Can you work these out from the model? Positions are in its coordinate system, mm. Give positions to 0.01 mm unless a question says otherwise; leave off trailing zeros. Loops run counter-clockwise (first coordinate to the right, second up) from the corner with the lowest first, then second, coordinate; pieces in that order, holes last. Notation, with made-up numbers: M 53,-29 L 73,-29 A30 cw 73,9 Z; hole C 73,-19 d3. An arc over 180 degrees is marked long. Answer as a JSON object with one key per item and string values.
```python
from build123d import *

# Parameters (mm, degrees)
CUT_EXTRUDE1_DEPTH     = 1.5625
CUT_SWEEP1_PITCH       = 0.8
CUT_SWEEP1_HEIGHT      = 6.05
CUT_SWEEP1_RADIUS      = 2.5
CUT_SWEEP1_START_ANGLE = -90


with BuildPart() as part:
    # Sketch2 → Revolve1 (revolve)
    with BuildSketch(Plane.XY, mode=Mode.PRIVATE) as revolve1_sk:
        Polygon((-4, 0), (-4, 1.75), (-1.25, 1.75), (-0.5, 2.5), (3.2, 2.5), (4, 1.7), (4, 0), align=None)
    revolve(revolve1_sk.sketch.rotate(Axis((-4, 0, 0), (1, 0, 0)), 90), axis=Axis((-4, 0, 0), (1, 0, 0)))

    # Sketch3 → Cut-Extrude1 (cut)
    with BuildSketch(Plane(origin=(4, 0, 0), x_dir=(0, 0, -1), z_dir=(1, 0, 0))):
        Polygon((0.721687836, 1.25), (-0.721687836, 1.25), (-1.443375673, 0), (-0.721687836, -1.25), (0.721687836, -1.25), (1.443375673, 0), align=None)
    extrude(amount=-CUT_EXTRUDE1_DEPTH, mode=Mode.SUBTRACT)

    # Cut-Extrude2 cone 1 section (through the dimple's axis) → Cut-Extrude2 (revolve, cut)
    with BuildSketch(Plane(origin=(4, 0, 0), x_dir=(0, 0, -1), z_dir=(0, 1, 0))):
        Polygon((0, 0), (1.443375673, 0), (0, 0.833333333), align=None)
    revolve(axis=Axis((4, 0, 0), (-1, 0, 0)), mode=Mode.SUBTRACT)

    # Cut-Extrude3 cone 1 section (through the dimple's axis) → Cut-Extrude3 (revolve, cut)
    with BuildSketch(Plane(origin=(2.4375, 0, 0), x_dir=(0, 0, -1), z_dir=(0, 1, 0))):
        Polygon((0, 0), (1.25, 0), (0, 0.721687836), align=None)
    revolve(axis=Axis((2.4375, 0, 0), (-1, 0, 0)), mode=Mode.SUBTRACT)

    # Cut-Sweep1: sweep along a helix
    with BuildLine() as cut_sweep1_path:
        add(Helix(CUT_SWEEP1_PITCH, CUT_SWEEP1_HEIGHT, CUT_SWEEP1_RADIUS, center=(4, 0, 0), direction=(-1, 0, 0), mode=Mode.PRIVATE).rotate(Axis((4, 0, 0), (-1, 0, 0)), CUT_SWEEP1_START_ANGLE))
    # Sketch6 → Cut-Sweep1 (sweep, cut)
    with BuildSketch(Plane.XY):
        Polygon((3.975, 2.54330127), (4.725, 2.54330127), (4.4, 1.980384758), (4.3, 1.980384758), align=None)
    sweep(path=cut_sweep1_path.line, is_frenet=True, mode=Mode.SUBTRACT)


solid = part.part
```
1) If we mould it in two halves opening along Y, with no side actions, what happens to faces 1 (the flat face through (-4, 0, 0)), 2 (the flat face through (3, -1.25, 0)), 3 (the cylindrical face through (-2.61, 1.55, 0.81))? For each: +Y half, -Y half, draft (parallel to the pull), parting line (faces both ways), or undercut.
Answer list:
{"face 1": "draft", "face 2": "undercut", "face 3": "parting line"}
2) Suppose I cut it at A-A, the plane x = -3. Write out the boundary of the cut face in (y, z).
Answer list:
{"outline": "C 0,0 d3.5"}
3) Will these pins go through, and if not, where does the flat tip stop? pin 1 Ø3 at (x, z) = (1.5, -2) entering from -Y; pin 2 Ø1.6 at (x, z) = (3.5, -0.5) entering from -Y; pin 3 Ø1.5 at (x, y) = (-2, -1.5) entering from +Z.
Answer list:
{"pin 1": "y = -2.44", "pin 2": "y = -2.5", "pin 3": "z = 1.58"}
4) Please list where these lines run through material, in increasing order: line 1 along Y through (x, z) = (3, -0.55); line 2 along X through (y, z) = (-0.8, 2); line 3 along Z through (x, y) = (2.75, 0.45). Write a range as from..to.
Answer list:
{"line 1": "-2.14..-1.25, 1.25..2.31", "line 2": "-0.85..-0.35, -0.05..0.45, 0.75..1.25, 1.55..2.05, 2.35..2.85, 3.15..3.55", "line 3": "-2.15..-1.18, 1.18..2.15"}
